Part model, mm, in its own coordinate system. A direction names the side the tool comes from. Round coordinates to 2 decimals unless told otherwise and drop trailing zeros. Order: outer loops, then holes, each group sorted by start corner. A loop starts at its lowest first (then second) coordinate and runs counter-clockwise, first axis right, second up. Notation, with made-up numbers: (-34, 84.5) - (0, 84.5) arc R11 cw to (0, 105.5) - close; hole circle Ø11 at (59.5, 18). An arc over 180 degrees is marked (long way). Return JSON: item names as keys, results as strings. Group by question number.
Item 1: Drop flat-ended pins along their axis: pin 1 (8 mm diameter, centred on x = -7.5, z = -16, fed in from +Y); pin 2 (11.5 mm diameter, centred on x = 5, z = 0, fed in from +Y); pin 3 (8 mm diameter, centred on y = 15, z = -9, fed in from +X); pin 4 (2 mm diameter, centred on y = 11, z = 9, fed in from -X). Give the stop position or say it passes through.
Item 2: Saw through at B-B on y = 2.5. List the corners of the cut face in (x, z), and give its area (3 significant figures).
Item 3: Two-plate mould, pull along Y, no slides. Class faces 1 (the face through (-8, 6, 24.194)), 2 (the face through (-6.6, 11.55, 34.6)), 3 (the face through (-11.684, 14, -34)): released by +Y, released by -Y, zero draft, split by the parting line, or undercut.
Item 4: Tool access for faces 4 (the face through (-8, 6, -24.194)), 5 (the face through (-5.375, 6.772, 24.998)), 6 (the face through (-4.526, 13, 0)): list every direction of +Z, -Z, +X, -X, +Y, -Y with a clear straight run to the whole face (end or side of a thin tool).
Item 5: Saw through at C-C on x = -3. List the corners of the cut face in (y, z).
Item 6: Probe probe 1 along Y at (x, z) = (16, -13); probe 2 along Y at (x, z) = (-5, 22); probe 3 along X at (y, z) = (13.5, -19). List the from-to ranges inside material, lowest first.
Item 7: Saw through at A-A on z = 16. List the corners of the cut face in (x, y).
Item 8: Saw through at D-D on y = 11.25. List the corners of the cut face in (x, z).
```python
from build123d import *

# Parameters (mm, degrees)
BOSS_EXTRUDE1_DEPTH = 1.5875
BOSS_EXTRUDE3_DEPTH = 1.5875
SKETCH9_W           = 7.115403393296309
SKETCH9_H           = 66.67028171012657
BOSS_EXTRUDE4_DEPTH = 1.5875
BOSS_EXTRUDE5_DEPTH = 1.5875
CHAMFER1_SIZE       = 0.6614583333333334
CHAMFER2_SIZE       = 0.6614583333333334
BOSS_EXTRUDE6_DEPTH = 1.5875
FILLET5_R           = 0.79375


with BuildPart() as part:
    # 3DSketch3 → Boss-Extrude1 (new body)
    with BuildSketch(Plane(origin=(11.684, 0, 25.781), x_dir=(-0.41278854058734626, 0, -0.910826888469905), z_dir=(0, 1, 0))):
        Polygon((0, 0), (9.646042616445111, 21.284202729764747), (56.61009863973035, 0), (46.96405602328524, -21.284202729764747), align=None)
    extrude(amount=BOSS_EXTRUDE1_DEPTH)

    # Sketch1 → Boss-Extrude3 (add)
    with BuildSketch(Plane.XY.offset(25.781)):
        Polygon((-3.47e-15, 0), (-10.08001412814663, 12.7), (-11.684000000000005, 12.7), (-11.684000000000005, 0), align=None)
    boss_extrude3 = extrude(amount=-BOSS_EXTRUDE3_DEPTH)

    # Mirror2: Boss-Extrude3 across plane
    add(boss_extrude3.mirror(Plane.XY))

    # Sketch9 → Boss-Extrude4 (add)
    with BuildSketch(Plane(origin=(0, 12.7, 0), x_dir=(1, 0, 0), z_dir=(0, 1, 0))):
        with Locations((-8.083759928300761, 0)):
            Rectangle(SKETCH9_W, SKETCH9_H)
    extrude(amount=BOSS_EXTRUDE4_DEPTH)

    # Sketch10 → Boss-Extrude5 (add)
    with BuildSketch(Plane.XY.offset(33.33514085506329)):
        Polygon((-11.684000000000005, 9.710531383967755), (-11.684000000000005, 18.08556377199017), (-1.4701183607090107, 18.08556377199017), (-1.4701183607090107, 12.7), align=None)
    boss_extrude5 = extrude(amount=BOSS_EXTRUDE5_DEPTH)

    # Chamfer1
    chamfer1_edges = [part.edges().sort_by_distance(p)[0] for p in [
        (-1.4701183607090107, 15.392781885995085, 33.33514085506329),
        (-6.5770591803545075, 11.205265691983877, 33.33514085506329),
        (-6.5770591803545075, 18.08556377199017, 33.33514085506329),
        (-1.4701183607090107, 15.392781885995085, 34.922640855063285),
        (-6.5770591803545075, 18.08556377199017, 34.922640855063285),
        (-6.5770591803545075, 11.205265691983877, 34.922640855063285),
    ]]
    chamfer(chamfer1_edges, length=CHAMFER1_SIZE)

    # Mirror4: Boss-Extrude5 across plane
    add(boss_extrude5.mirror(Plane.XY))

    # Chamfer2
    chamfer2_edges = [part.edges().sort_by_distance(p)[0] for p in [
        (-1.4701183607090107, 15.392781885995085, -33.33514085506329),
        (-6.5770591803545075, 11.205265691983877, -33.33514085506329),
        (-6.5770591803545075, 18.08556377199017, -33.33514085506329),
        (-1.4701183607090107, 15.392781885995085, -34.922640855063285),
        (-6.5770591803545075, 11.205265691983877, -34.922640855063285),
        (-6.5770591803545075, 18.08556377199017, -34.922640855063285),
    ]]
    chamfer(chamfer2_edges, length=CHAMFER2_SIZE)

    # Sketch12 → Boss-Extrude6 (add)
    with BuildSketch(Plane(origin=(0, 0, 0), x_dir=(1, 0, 0), z_dir=(0, 1, 0))):
        Polygon((11.684, 25.781), (27.685999999999996, 25.781), (27.686000000000003, -25.810245145350073), (11.684, -25.810245145350073), align=None)
    extrude(amount=BOSS_EXTRUDE6_DEPTH)

    # Fillet5
    fillet5_edges = [part.edges().sort_by_distance(p)[0] for p in [
        (19.685000000000002, 1.5875, 25.810245145350073),
        (13.212999116990831, 1.5875, -25.781),
        (27.686, 1.5875, 0.0146225726750373),
    ]]
    fillet(fillet5_edges, radius=FILLET5_R)


solid = part.part
```
Filled in:
{
 "1": {"pin 1": "stops at y = 14.29", "pin 2": "stops at y = 1.59", "pin 3": "stops at x = -4.53", "pin 4": "passes through"},
 "2": {"outline": "(-11.68, -25.78) - (-1.98, -25.78) - (-1.98, -24.19) - (-11.68, -24.19) - close; (-11.68, 24.19) - (-1.98, 24.19) - (-1.98, 25.78) - (-11.68, 25.78) - close", "area": "30.8 mm^2"},
 "3": {"face 1": "undercut", "face 2": "released by -Y", "face 3": "zero draft"},
 "4": {"face 4": "+X, -X", "face 5": "+X", "face 6": "+X, +Y"},
 "5": {"outline": "(0, -25.78) - (3.78, -25.78) - (3.78, -24.19) - (1.59, -24.19) - (1.59, 24.19) - (3.78, 24.19) - (3.78, 25.78) - (0, 25.78) - close; (12.25, -34.26) - (12.94, -34.92) - (17.42, -34.92) - (18.09, -34.26) - (18.09, -34) - (17.42, -33.34) - (12.94, -33.34) - (12.25, -34) - close; (12.25, 34) - (12.94, 33.34) - (17.42, 33.34) - (18.09, 34) - (18.09, 34.26) - (17.42, 34.92) - (12.94, 34.92) - (12.25, 34.26) - close"},
 "6": {"probe 1": "y = 0 to 1.59", "probe 2": "y = 0 to 1.59, 12.7 to 14.29", "probe 3": "x = -11.64 to -4.53"},
 "7": {"outline": "(-11.68, 0) - (27.69, 0) - (27.69, 0.79) arc R0.79 ccw to (26.89, 1.59) - (-11.68, 1.59) - close; (-11.64, 12.7) - (-4.53, 12.7) - (-4.53, 14.29) - (-11.64, 14.29) - close"},
 "8": {"outline": "(-11.68, -34.92) - (-8.78, -34.92) - (-6.42, -34.26) - (-6.42, -34) - (-8.78, -33.34) - (-11.68, -33.34) - close; (-11.68, -25.78) - (-8.93, -25.78) - (-8.93, -24.19) - (-11.68, -24.19) - close; (-11.68, 24.19) - (-8.93, 24.19) - (-8.93, 25.78) - (-11.68, 25.78) - close; (-11.68, 33.34) - (-8.78, 33.34) - (-6.42, 34) - (-6.42, 34.26) - (-8.78, 34.92) - (-11.68, 34.92) - close"}
}
